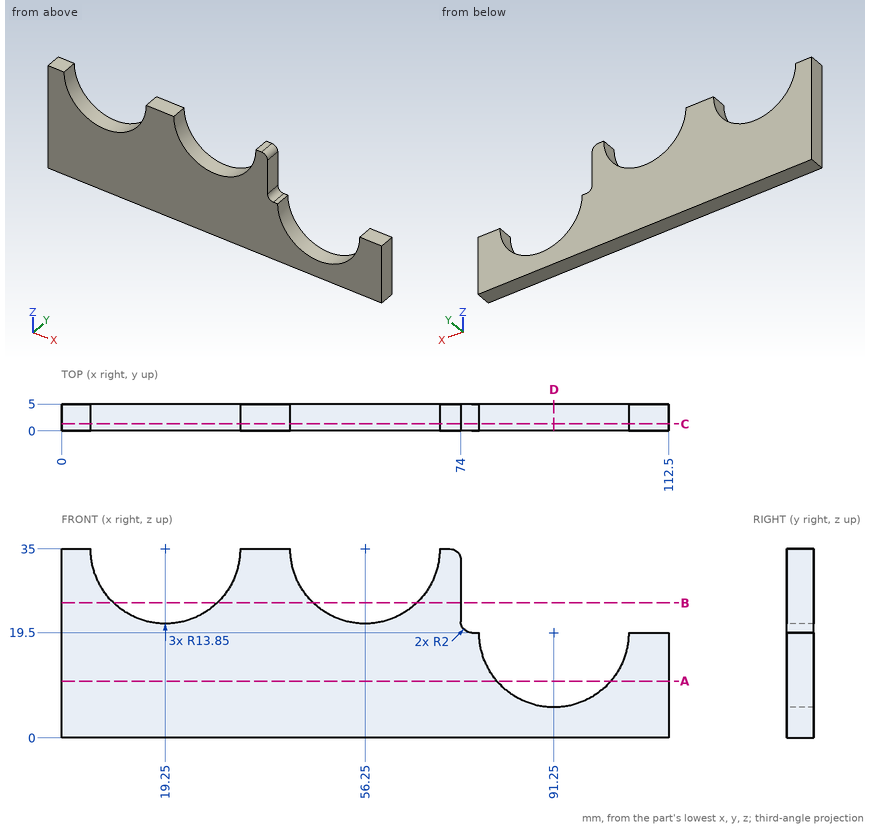
Here's the drawing with two shaded views (mm, measured from the low corner). I have some questions. Round coordinates to 2 decimals unless told otherwise and drop trailing zeros. Order: outer loops, then holes, each group sorted by start corner. A loop starts at its lowest first (then second) coordinate and runs counter-clockwise, first axis right, second up. Notation, with made-up numbers: (52.25, -11) -> (61.25, -11) arc R16 cw to (61.25, -4) -> close; hole circle Ø3 at (54.25, -1). An arc over 180 degrees is marked (long way). Return JSON: item names as keys, results as strings.
Q1. If we section it at D-D on x = 91.25: List the corners of the cut face in (y, z) for me, plus the area to 4 significant figures.
Filled sheet:
{"outline": "(0, 0) -> (5, 0) -> (5, 5.65) -> (0, 5.65) -> close", "area": "28.25 mm^2"}
Q2. I need wall thicknesses on line 1 along X through (y, z) = (2.9, 23); line 2 along X through (y, z) = (2.25, 25.5); line 3 along X through (y, z) = (4.2, 17). Which ranges of each line are inside material? Lowest first, please. Write a range as from..to.
Filled sheet:
{"line 1": "x = 0..12.33, 26.17..49.33, 63.17..74", "line 2": "x = 0..9.17, 29.33..46.17, 66.33..74", "line 3": "x = 0..77.63, 104.87..112.5"}
Q3. If we section it at A-A on z = 10.5: List the corners of the cut face in (x, y) for me.
Filled sheet:
{"outline": "(0, 0) -> (80.72, 0) -> (80.72, 5) -> (0, 5) -> close; (101.78, 0) -> (112.5, 0) -> (112.5, 5) -> (101.78, 5) -> close"}
Q4. For pin 1 Ø0.7 at (x, y) = (77, 2.5) entering from +Z; pin 2 Ø1 at (x, y) = (32.5, 3.5) entering from -Z; pin 3 Ø2.5 at (y, z) = (2.5, 30) entering from +X, each with a flat end and sliding along its axis, tell me the tip position at first contact or that it passes through.
Filled sheet:
{"pin 1": "stops at z = 19.5", "pin 2": "stops at z = 0", "pin 3": "stops at x = 74"}
Q5. If we section it at C-C on y = 1.3: List the corners of the cut face in (x, z) for me, plus the area to 3 significant figures.
Filled sheet:
{"outline": "(0, 0) -> (112.5, 0) -> (112.5, 19.5) -> (105.1, 19.5) arc R13.85 cw to (77.4, 19.5) -> (76, 19.5) arc R2 cw to (74, 21.5) -> (74, 33) arc R2 ccw to (72, 35) -> (70.1, 35) arc R13.85 cw to (42.4, 35) -> (33.1, 35) arc R13.85 cw to (5.4, 35) -> (0, 35) -> close", "area": "2,440 mm^2"}
Q6. If we section it at B-B on z = 25: List the corners of the cut face in (x, y) for me, plus the area to 3 significant figures.
Filled sheet:
{"outline": "(0, 0) -> (9.67, 0) -> (9.67, 5) -> (0, 5) -> close; (28.83, 0) -> (46.67, 0) -> (46.67, 5) -> (28.83, 5) -> close; (65.83, 0) -> (74, 0) -> (74, 5) -> (65.83, 5) -> close", "area": "178 mm^2"}
